CAD build for the part. Positions are in the model's coordinates, mm. Coordinates: 2 decimals unless noted, no trailing zeros. Loops run counter-clockwise (first coordinate to the right, second up) from the corner with the lowest first, then second, coordinate; pieces in that order, holes last. Notation, with made-up numbers: (-23.75, 32) -> (-3.75, 32) arc R19 cw to (-3.75, 67) -> close; hole circle Ø8 at (55.5, 8). An arc over 180 degrees is marked (long way). Return JSON: item names as keys, results as strings. Group by question number.
(1) Probe L1, parallel to X at y = 3, z = -4; L2, parallel to Z at x = 0, y = 4.45; L3, parallel to Z at x = 0.5, y = 1.6. List the from-to ranges inside material, lowest first.
(2) Mould opens along X. For faces 1 (the face through (23.5, 3, -4)), 2 (the face through (0, 3, 0)), 3 (the face through (-0.325, 2.958, -12.536)) say: pulls with the +X half, pulls with the -X half, needs draft (parallel to the pull), parting line crosses it, or undercut.
(3) Saw through at C-C on z = -4. Write the cut outline in (x, y), then the cut area to 3 significant figures.
(4) Saw through at A-A on y = 0.8. Write the cut outline in (x, z), then the cut area to 3 significant figures.
(5) Flat gauge pins, fed straight in: pin 1 Ø5 at (x, z) = (0, -4) entering from +Y (3 decimals); pin 2 Ø1 at (x, y) = (13.5, 4) entering from -Z; pin 3 Ø2 at (y, z) = (3, -13) entering from +X; pin 4 Ø4 at (x, z) = (20, -4) entering from -Y. Where does each tip first touch, or does it go through?
(6) Saw through at B-B on x = 0. Write the cut outline in (y, z), then the cut area to 3 significant figures.
(7) Saw through at D-D on x = 20. Write the cut outline in (y, z).
```python
from build123d import *

# Parameters (mm, degrees)
SKETCH1_R           = 3
SKETCH1_R_2         = 1.5
BOSS_EXTRUDE1_DEPTH = 6
FILLET1_R           = 3


with BuildPart() as part:
    # Sketch1 → Boss-Extrude1 (new body)
    with BuildSketch(Plane(origin=(0, 0, 0), x_dir=(1, 0, 0), z_dir=(0, 1, 0))):
        Polygon((23.5, 0), (-23.5, 0), (-23.5, 6.946022727), (0, 17.5), (23.5, 6.946022727), align=None)
        with Locations((0, 4)):
            Circle(SKETCH1_R, mode=Mode.SUBTRACT)
        with Locations((20, 4)):
            Circle(SKETCH1_R_2, mode=Mode.SUBTRACT)
        with Locations((-20, 4)):
            Circle(SKETCH1_R_2, mode=Mode.SUBTRACT)
        with Locations((0, 14)):
            Circle(SKETCH1_R_2, mode=Mode.SUBTRACT)
    extrude(amount=BOSS_EXTRUDE1_DEPTH)

    # Fillet1
    fillet1_edges = [part.edges().sort_by_distance(p)[0] for p in [
        (23.5, 3, 0),
        (-23.5, 3, 0),
        (-23.5, 3, -6.946022727),
        (0, 3, -17.5),
        (23.5, 3, -6.946022727),
    ]]
    fillet(fillet1_edges, radius=FILLET1_R)


solid = part.part
```
Geometry results:
{
 "1": {"L1": "-23.5 to -21.5, -18.5 to -3, 3 to 18.5, 21.5 to 23.5", "L2": "-17.21 to -15.5, -12.5 to -7, -1 to 0", "L3": "-17.17 to -15.41, -12.59 to -6.96, -1.04 to 0"},
 "2": {"face 1": "pulls with the +X half", "face 2": "needs draft", "face 3": "undercut"},
 "3": {"outline": "(-23.5, 0) -> (-21.5, 0) -> (-21.5, 6) -> (-23.5, 6) -> close; (-18.5, 0) -> (-3, 0) -> (-3, 6) -> (-18.5, 6) -> close; (3, 0) -> (18.5, 0) -> (18.5, 6) -> (3, 6) -> close; (21.5, 0) -> (23.5, 0) -> (23.5, 6) -> (21.5, 6) -> close", "area": "210 mm²"},
 "4": {"outline": "(-23.5, -5) arc R3 ccw to (-21.73, -7.74) -> (-1.23, -16.95) arc R3 ccw to (1.23, -16.95) -> (21.73, -7.74) arc R3 ccw to (23.5, -5) -> (23.5, -3) arc R3 ccw to (20.5, 0) -> (-20.5, 0) arc R3 ccw to (-23.5, -3) -> close; hole circle Ø3 at (-20, -4); hole circle Ø6 at (0, -4); hole circle Ø3 at (0, -14); hole circle Ø3 at (20, -4)", "area": "520 mm²"},
 "5": {"pin 1": "through", "pin 2": "z = -11.66", "pin 3": "x = 12.25", "pin 4": "y = 0"},
 "6": {"outline": "(0, -17.21) -> (6, -17.21) -> (6, -15.5) -> (0, -15.5) -> close; (0, -12.5) -> (6, -12.5) -> (6, -7) -> (0, -7) -> close; (0, -1) -> (6, -1) -> (6, 0) -> (0, 0) -> close", "area": "49.3 mm²"},
 "7": {"outline": "(0, -8.52) -> (6, -8.52) -> (6, -5.5) -> (0, -5.5) -> close; (0, -2.5) -> (6, -2.5) -> (6, 0) -> (0, 0) -> close"}
}
